Geometry check sheet. Reference: the model listing, model coordinates, mm. A direction names the side the tool comes from. Round coordinates to 2 decimals unless told otherwise and drop trailing zeros. Order: outer loops, then holes, each group sorted by start corner. A loop starts at its lowest first (then second) coordinate and runs counter-clockwise, first axis right, second up.
(1) Draft check along Y on faces 3 (the face through (98.78, 220.21, 3.22)), 4 (the face through (63, 0, 3)), 5 (the face through (47.625, 101, 3)), 6 (the face through (63, 126, 6.35)). Enter one of: pulls with the +Y half, pulls with the -Y half, needs draft (parallel to the pull), parting line crosses it, or undercut.
(2) Cross-section at D-D on x = 29. Enter the section's corners in (y, z), and give its area (3 significant figures).
(3) Set-up check for faces 1 (the face through (111.125, 101, 3)), 2 (the face through (0, 106, 3)): record each of +Z, -Z, +X, -X, +Y, -Y from which the full face is reachable in a straight line by a thin tool's end or side.
(4) Cross-section at B-B on y = 122. Enter the section's corners in (x, z) (3 decimals).
(5) Gauge pin test, flat end, axial feed: P1, Ø2, axis at x = 62, z = 4, coming from the +Y side. Record the tip position at first contact, or that the pin passes through.
(6) Cross-section at A-A on z = 3. Enter the section's corners in (x, y) (3 decimals), and give its area (3 significant figures).
(7) Thickness scan on L1, parallel to X at y = 92.5, z = 5.5 (3 decimals); L2, parallel to Y at x = 21.5, z = 5.5; L3, parallel to Y at x = 84.5, z = 6. Record the ranges inside material, lowest first.
(8) Cross-section at C-C on x = 93.5. Enter the section's corners in (y, z), and give its area (3 significant figures).
from build123d import *

# Parameters (mm, degrees)
SKETCH1_W           = 127
SKETCH1_H           = 247.65
BOSS_EXTRUDE1_DEPTH = 6.35
CUT_EXTRUDE1_DEPTH  = 279.387939753
SKETCH3_W           = 31.75
SKETCH3_H           = 152.4
CUT_EXTRUDE2_DEPTH  = 279.387939753


with BuildPart() as part:
    # Sketch1 → Boss-Extrude1 (new body)
    with BuildSketch(Plane.XY):
        with Locations((63.5, 123.825)):
            Rectangle(SKETCH1_W, SKETCH1_H)
    extrude(amount=BOSS_EXTRUDE1_DEPTH)

    # Sketch2 → Cut-Extrude1 (cut, through all)
    with BuildSketch(Plane.XY.offset(6.35)):
        Polygon((0, 214.383772574), (71.339654933, 247.65), (0, 247.65), align=None)
        Polygon((127, 247.65), (71.339654933, 247.65), (127, 191.989654933), align=None)
    extrude(amount=-CUT_EXTRUDE1_DEPTH, mode=Mode.SUBTRACT)

    # Sketch3 → Cut-Extrude2 (cut, through all)
    with BuildSketch(Plane.XY.offset(6.35)):
        with Locations((31.75, 101.6)):
            Rectangle(SKETCH3_W, SKETCH3_H)
        with Locations((95.25, 101.6)):
            Rectangle(SKETCH3_W, SKETCH3_H)
    extrude(amount=-CUT_EXTRUDE2_DEPTH, mode=Mode.SUBTRACT)


solid = part.part
Found:
1. face 3: pulls with the +Y half
1. face 4: pulls with the -Y half
1. face 5: undercut
1. face 6: needs draft
2. outline: (0, 0) - (25.4, 0) - (25.4, 6.35) - (0, 6.35) - close; (177.8, 0) - (227.91, 0) - (227.91, 6.35) - (177.8, 6.35) - close
2. area: 479 mm2
3. face 1: +Z, -Z
3. face 2: +Z, -Z, -X, +Y, -Y
4. outline: (0, 0) - (15.875, 0) - (15.875, 6.35) - (0, 6.35) - close; (47.625, 0) - (79.375, 0) - (79.375, 6.35) - (47.625, 6.35) - close; (111.125, 0) - (127, 0) - (127, 6.35) - (111.125, 6.35) - close
5. P1: stops at y = 243.76
6. outline: (0, 0) - (127, 0) - (127, 191.99) - (71.34, 247.65) - (0, 214.384) - close; hole (15.875, 25.4) - (47.625, 25.4) - (47.625, 177.8) - (15.875, 177.8) - close; hole (79.375, 25.4) - (111.125, 25.4) - (111.125, 177.8) - (79.375, 177.8) - close
6. area: 19,000 mm2
7. L1: x = 0 to 15.875, 47.625 to 79.375, 111.125 to 127
7. L2: y = 0 to 25.4, 177.8 to 224.41
7. L3: y = 0 to 25.4, 177.8 to 234.49
8. outline: (0, 0) - (25.4, 0) - (25.4, 6.35) - (0, 6.35) - close; (177.8, 0) - (225.49, 0) - (225.49, 6.35) - (177.8, 6.35) - close
8. area: 464 mm2
